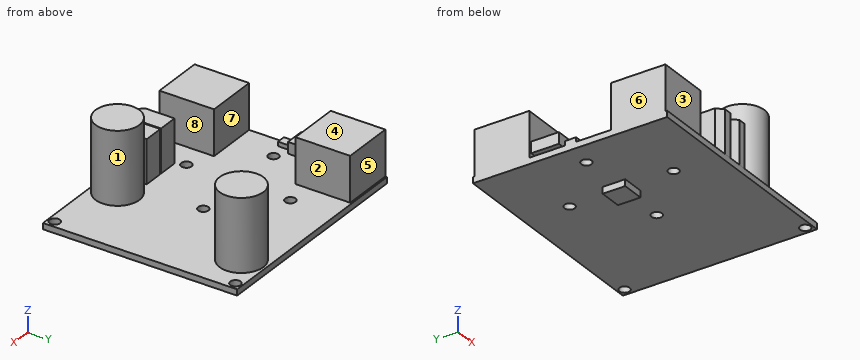
```python
from build123d import *

# Parameters (mm, degrees)
SKETCH1_W                 = 64
SKETCH1_H                 = 56
BOSS_EXTRUDE1_DEPTH       = 1.75
SKETCH2_W                 = 5.6
SKETCH2_H                 = 8
BOSS_EXTRUDE2_DEPTH       = 3.249999999
BOSS_EXTRUDE3_DEPTH       = 12.5
SKETCH4_W                 = 2.5
SKETCH4_H                 = 3.249999996
BOSS_EXTRUDE4_DEPTH       = 1.250000001
SKETCH5_W                 = 15
SKETCH5_H                 = 15.750000006
BOSS_EXTRUDE5_DEPTH       = 12.999999998
SKETCH6_W                 = 15
SKETCH6_H                 = 15.749999994
BOSS_EXTRUDE6_DEPTH       = 13
BOSS_EXTRUDE7_DEPTH       = 12.5
SKETCH8_W                 = 6.5
SKETCH8_H                 = 6.499999992
BOSS_EXTRUDE8_DEPTH       = 1.9
SKETCH9_W                 = 6.325
SKETCH9_H                 = 20.8
SKETCH10_W                = 6.325
SKETCH10_H                = 20.8
F_3_CLEARANCE_HOLE1_D     = 3
F_3_CLEARANCE_HOLE1_DEPTH = 22.55


with BuildPart() as part:
    # Sketch1 → Boss-Extrude1 (new body)
    with BuildSketch(Plane(origin=(0, 0, 9.525), x_dir=(-1, 0, 0), z_dir=(0, 0, -1))):
        with Locations((-70.325, 0)):
            Rectangle(SKETCH1_W, SKETCH1_H)
    extrude(amount=-BOSS_EXTRUDE1_DEPTH)

    # Sketch2 → Boss-Extrude2 (add)
    with BuildSketch(Plane.XY.offset(11.275)):
        with Locations((39.625, 6.2)):
            Rectangle(SKETCH2_W, SKETCH2_H)
    extrude(amount=BOSS_EXTRUDE2_DEPTH)

    # Sketch3 → Boss-Extrude3 (add)
    with BuildSketch(Plane.XY.offset(11.275)):
        Polygon((61.45, -17.675), (67.199999996, -17.675), (67.199999996, -26.174999992), (65.449999996, -27.924999992), (63.2, -27.924999992), (61.45, -26.174999992), align=None)
    extrude(amount=BOSS_EXTRUDE3_DEPTH)

    # Sketch4 → Boss-Extrude4 (add)
    with BuildSketch(Plane.XY.offset(11.275)):
        with Locations((39.575, -0.125000002)):
            Rectangle(SKETCH4_W, SKETCH4_H)
    extrude(amount=BOSS_EXTRUDE4_DEPTH)

    # Sketch5 → Boss-Extrude5 (add)
    with BuildSketch(Plane.XY.offset(11.275)):
        with Locations((45.825, -19.625000009)):
            Rectangle(SKETCH5_W, SKETCH5_H)
    extrude(amount=BOSS_EXTRUDE5_DEPTH)

    # Sketch6 → Boss-Extrude6 (add)
    with BuildSketch(Plane.XY.offset(11.275)):
        with Locations((45.825, 19.625000009)):
            Rectangle(SKETCH6_W, SKETCH6_H)
    extrude(amount=BOSS_EXTRUDE6_DEPTH)

    # Sketch7 → Boss-Extrude7 (add)
    with BuildSketch(Plane.XY.offset(11.275)):
        Polygon((67.55, -17.675), (73.299999996, -17.675), (73.299999996, -26.174999992), (71.549999996, -27.924999992), (69.3, -27.924999992), (67.55, -26.174999992), align=None)
    extrude(amount=BOSS_EXTRUDE7_DEPTH)

    # Sketch8 → Boss-Extrude8 (add)
    with BuildSketch(Plane(origin=(0, 0, 9.525), x_dir=(-1, 0, 0), z_dir=(0, 0, -1))):
        with Locations((-60.325, 0)):
            Rectangle(SKETCH8_W, SKETCH8_H)
    extrude(amount=BOSS_EXTRUDE8_DEPTH)

    # Sketch9 → Revolve1 (revolve)
    with BuildSketch(Plane.XZ.offset(21.3)):
        with Locations((83.5875, 21.675)):
            Rectangle(SKETCH9_W, SKETCH9_H)
    revolve(axis=Axis((80.425, -21.3, 32.075), (0, 0, -1)))

    # Sketch10 → Revolve2 (revolve)
    with BuildSketch(Plane.XZ.offset(-21)):
        with Locations((93.2875, 21.675)):
            Rectangle(SKETCH10_W, SKETCH10_H)
    revolve(axis=Axis((90.125, 21, 32.075), (0, 0, -1)))

    # #3 Clearance Hole1
    with Locations(Plane(origin=(0, 0, 9.525), x_dir=(-1, 0, 0), z_dir=(0, 0, -1))):
        with Locations((-45.325, 0), (-60.325, 15), (-75.325, 0), (-60.325, -15), (-100.175, 26.05), (-100.175, -26.05)):
            Hole(F_3_CLEARANCE_HOLE1_D / 2, depth=F_3_CLEARANCE_HOLE1_DEPTH)


solid = part.part
```
Source: CAD feature listing. Evaluate the final solid. Frame: model axes, mm. Face numbers are marked on the shaded views. A direction names the side the tool comes from. Give positions to 0.01 mm unless a question says otherwise; leave off trailing zeros. Order: outer loops, then holes, each group sorted by start corner. A loop starts at its lowest first (then second) coordinate and runs counter-clockwise, first axis right, second up. Notation, with made-up numbers: (7.5, 20.5) -> (65.5, 20.5) arc R24 ccw to (65.5, 47.5) -> close; hole circle Ø5 at (-7.5, -23.75). An arc over 180 degrees is marked (long way). Use a Markdown table: item, result.
Q1. Material intervals for line 1 (X direction, y = -21, z = 22.5) (3 decimals); line 2 (Y direction, x = 52.5, z = 12.75); line 3 (Z direction, x = 97.5, y = 0.5) (3 decimals), sorted ascending. Write a range as [from, to].
A:
| item | result |
|---|---|
| line 1 | [38.325, 53.325], [61.45, 67.2], [67.55, 73.3], [74.107, 86.743] |
| line 2 | [-27.5, -11.75], [11.75, 27.5] |
| line 3 | [9.525, 11.275] |
Q2. Access query for the marked faces 1, 2, 3, 4 and 5. Directions: +Z, -Z, +X, -X, +Y, -Y. A direction counts if a zero-diameter tool reaches every point of the face in a straight line with its end or side. Return the directions, or none.
A:
| item | result |
|---|---|
| face 1 | +Z |
| face 2 | +Z, +Y, -Y |
| face 3 | +Z, -X, -Y |
| face 4 | +Z, -X, +Y, -Y |
| face 5 | +Z, +X, -X, +Y |
Q3. Section B-B (y = 26.05). Return the cut outline in (x, z) (3 decimals).
A:
| item | result |
|---|---|
| outline | (38.325, 9.525) -> (98.675, 9.525) -> (98.675, 11.275) -> (93.933, 11.275) -> (93.933, 32.075) -> (86.317, 32.075) -> (86.317, 11.275) -> (53.325, 11.275) -> (53.325, 24.275) -> (38.325, 24.275) -> close; (101.675, 9.525) -> (102.325, 9.525) -> (102.325, 11.275) -> (101.675, 11.275) -> close |
Q4. Section A-A (z = 16). Return the cut outline in (x, y) (3 decimals).
A:
| item | result |
|---|---|
| outline | (38.325, -27.5) -> (53.325, -27.5) -> (53.325, -11.75) -> (38.325, -11.75) -> close; (38.325, 11.75) -> (53.325, 11.75) -> (53.325, 27.5) -> (38.325, 27.5) -> close; (61.45, -26.175) -> (63.2, -27.925) -> (65.45, -27.925) -> (67.2, -26.175) -> (67.2, -17.675) -> (61.45, -17.675) -> close; (67.55, -26.175) -> (69.3, -27.925) -> (71.55, -27.925) -> (73.3, -26.175) -> (73.3, -17.675) -> (67.55, -17.675) -> close; circle Ø12.65 at (80.425, -21.3); circle Ø12.65 at (90.125, 21) |
Q5. Section D-D (x = 50). Return the cut outline in (y, z) (3 decimals), and give its area (4 significant figures).
A:
| item | result |
|---|---|
| outline | (-28, 9.525) -> (28, 9.525) -> (28, 11.275) -> (27.5, 11.275) -> (27.5, 24.275) -> (11.75, 24.275) -> (11.75, 11.275) -> (-11.75, 11.275) -> (-11.75, 24.275) -> (-27.5, 24.275) -> (-27.5, 11.275) -> (-28, 11.275) -> close |
| area | 507.5 mm^2 |
Q6. First-contact query: P1, Ø4, axis at x = 71.5, y = -20.5, coming from the -Z side (3 decimals); P2, Ø5, axis at y = -16, z = 15, coming from the +X side; P3, Ø1.7, axis at x = 71, y = -24, coming from the +Z side (3 decimals); P4, Ø0.6, axis at y = 0, z = 11.5, coming from the +X side (3 decimals). Flat tips, straight axial feed; report the tip coordinate or a pass-through.
A:
| item | result |
|---|---|
| P1 | z = 9.525 |
| P2 | x = 86.1 |
| P3 | z = 23.775 |
| P4 | x = 102.325 |
Q7. Section C-C (y = -21.3). Return the cut outline in (x, z) (3 decimals).
A:
| item | result |
|---|---|
| outline | (38.325, 9.525) -> (102.325, 9.525) -> (102.325, 11.275) -> (86.75, 11.275) -> (86.75, 32.075) -> (74.1, 32.075) -> (74.1, 11.275) -> (73.3, 11.275) -> (73.3, 23.775) -> (67.55, 23.775) -> (67.55, 11.275) -> (67.2, 11.275) -> (67.2, 23.775) -> (61.45, 23.775) -> (61.45, 11.275) -> (53.325, 11.275) -> (53.325, 24.275) -> (38.325, 24.275) -> close |
Q8. Pull-direction query (X, two-part tool) for the marked faces 6, 7 and 8; classes: +X half, -X half, draft (parallel to the pull), parting line (faces both ways), or undercut.
A:
| item | result |
|---|---|
| face 6 | -X half |
| face 7 | draft |
| face 8 | undercut |
